Verification items for the finished model (mm, model axes). A direction names the side the tool comes from. Coordinates: 2 decimals unless noted, no trailing zeros. Order: outer loops, then holes, each group sorted by start corner. A loop starts at its lowest first (then second) coordinate and runs counter-clockwise, first axis right, second up. Notation, with made-up numbers: M 75.5,85.25 L 100.5,85.25 A19 ccw 100.5,109.25 Z; hole C -7.75,89 d2. An arc over 180 degrees is marked long. Answer as a JSON object with one key per item and string values. Group by question number.
(1) Gauge pin test, flat ends, axial feed: pin 1 Ø1 at (y, z) = (11.5, 4.5) entering from -X; pin 2 Ø3 at (x, z) = (0, 10) entering from +Y; pin 3 Ø6 at (x, y) = (-15.5, 15.5) entering from -Z; pin 4 Ø6 at (y, z) = (5.5, 11) entering from +X. Record the tip position at first contact, or that the pin passes through.
(2) Mould release check, pull along Z, two halves, no side actions. Record for faces 1 (the face through (-5, -12, 20)), 2 (the face through (14, -17, 7.5)), 3 (the face through (19.2, 0.4, 8.4)), 4 (the face through (17.07, -16.15, 13.84)): released by +Z, released by -Z, zero draft, split by the parting line, or undercut.
(3) Access from +Z, -Z, +X, -X, +Y, -Y to the whole of each face (thin tool, end or side, straight path). Record for faces 5 (the face through (0, -20, 2)), 6 (the face through (-0.4, 19.4, 11.6)).
(4) Cross-section at B-B (z = 10). Enter the section's corners in (x, y).
(5) Material ranges on line 1 (Z direction, x = 22.25, y = 0); line 2 (Y direction, x = -15, z = 15.75); line 3 (Y direction, x = -15.5, z = 11.75), recorded low to high.
(6) Cross-section at A-A (x = 0). Enter the section's corners in (y, z), plus the area to 3 significant figures.
(7) Cross-section at C-C (x = -6). Enter the section's corners in (y, z), plus the area to 3 significant figures.
(8) Cross-section at D-D (z = 15.75). Enter the section's corners in (x, y).
from build123d import *

# Parameters (mm, degrees)
SKETCH1_W                                           = 26
SKETCH1_H                                           = 20
F_2_CLEARANCE_HOLE1_D                               = 2.5
F_2_CLEARANCE_HOLE1_DEPTH                           = 6
HOLE1_D                                             = 25.4
HOLE1_DEPTH                                         = 20
HOLE1_CBORE_D                                       = 40
HOLE1_CBORE_DEPTH                                   = 3.4
F_4_CLEARANCE_HOLE1_D                               = 3.3
F_4_CLEARANCE_HOLE1_DEPTH                           = 65.407641206
F_4_CLEARANCE_HOLE2_D                               = 3.3
F_4_CLEARANCE_HOLE2_DEPTH                           = 13.407641206
F_4_CLEARANCE_HOLE3_D                               = 3.3
F_4_CLEARANCE_HOLE3_DEPTH                           = 13.407641206
CBORE_FOR_4_BINDING_HEAD_MACHINE_SCREW1_D           = 3.4
CBORE_FOR_4_BINDING_HEAD_MACHINE_SCREW1_DEPTH       = 20
CBORE_FOR_4_BINDING_HEAD_MACHINE_SCREW1_CBORE_D     = 6.5
CBORE_FOR_4_BINDING_HEAD_MACHINE_SCREW1_CBORE_DEPTH = 7.5


with BuildPart() as part:
    # Sketch1 → Revolve1 (revolve)
    with BuildSketch(Plane.XZ):
        with Locations((13, 10)):
            Rectangle(SKETCH1_W, SKETCH1_H)
    revolve(axis=Axis((0, 0, 20), (0, 0, -1)))

    # #2 Clearance Hole1
    with Locations(Plane(origin=(0, 0, 0), x_dir=(-1, 0, 0), z_dir=(0, 0, -1))):
        with Locations((-22.776165581, 3.200981322)):
            Hole(F_2_CLEARANCE_HOLE1_D / 2, depth=F_2_CLEARANCE_HOLE1_DEPTH)

    # Hole1
    with Locations(Plane(origin=(0, 0, 0), x_dir=(-1, 0, 0), z_dir=(0, 0, -1))):
        with Locations((0, 0)):
            CounterBoreHole(HOLE1_D / 2, HOLE1_CBORE_D / 2, HOLE1_CBORE_DEPTH, depth=HOLE1_DEPTH)

    # #4 Clearance Hole1
    with Locations(Plane(origin=(26, 0, 10), x_dir=(0, 1, 0), z_dir=(1, 0, 0))):
        with Locations((0, 0)):
            Hole(F_4_CLEARANCE_HOLE1_D / 2, depth=F_4_CLEARANCE_HOLE1_DEPTH)

    # #4 Clearance Hole2
    with Locations(Plane(origin=(0, 12.592358794, 0), x_dir=(-1, 0, 0), z_dir=(0, -1, 0))):
        with Locations((0, -10)):
            Hole(F_4_CLEARANCE_HOLE2_D / 2, depth=F_4_CLEARANCE_HOLE2_DEPTH)

    # #4 Clearance Hole3
    with Locations(Plane(origin=(0, -12.592358794, 0), x_dir=(1, 0, 0), z_dir=(0, 1, 0))):
        with Locations((0, -10)):
            Hole(F_4_CLEARANCE_HOLE3_D / 2, depth=F_4_CLEARANCE_HOLE3_DEPTH)

    # CBORE for #4 Binding Head Machine Screw1
    with Locations(Plane(origin=(0, 0, 0), x_dir=(-1, 0, 0), z_dir=(0, 0, -1))):
        with Locations((-15.5, -15.5), (15.5, -15.5), (15.5, 15.5), (-15.5, 15.5)):
            CounterBoreHole(CBORE_FOR_4_BINDING_HEAD_MACHINE_SCREW1_D / 2, CBORE_FOR_4_BINDING_HEAD_MACHINE_SCREW1_CBORE_D / 2, CBORE_FOR_4_BINDING_HEAD_MACHINE_SCREW1_CBORE_DEPTH, depth=CBORE_FOR_4_BINDING_HEAD_MACHINE_SCREW1_DEPTH)


solid = part.part
Taken from the geometry:
{
 "1": {"pin 1": "stops at x = -23.56", "pin 2": "passes through", "pin 3": "stops at z = 7.5", "pin 4": "stops at x = 25.88"},
 "2": {"face 1": "released by +Z", "face 2": "released by -Z", "face 3": "undercut", "face 4": "zero draft"},
 "3": {"face 5": "-Z", "face 6": "+Y, -Y"},
 "4": {"outline": "M -25.95,-1.65 A26 ccw -1.65,-25.95 L -1.65,-12.59 A12.7 cw -12.59,-1.65 Z; M -25.95,1.65 L -12.59,1.65 A12.7 cw -1.65,12.59 L -1.65,25.95 A26 ccw Z; M 1.65,-25.95 A26 ccw 25.95,-1.65 L 12.59,-1.65 A12.7 cw 1.65,-12.59 Z; M 1.65,12.59 A12.7 cw 12.59,1.65 L 25.95,1.65 A26 ccw 1.65,25.95 Z; hole C -15.5,-15.5 d3.4; hole C -15.5,15.5 d3.4; hole C 15.5,-15.5 d3.4; hole C 15.5,15.5 d3.4"},
 "5": {"line 1": "z = 0 to 8.35, 11.65 to 20", "line 2": "y = -21.24 to -17.12, -13.88 to 13.88, 17.12 to 21.24", "line 3": "y = -20.87 to -17.2, -13.8 to 13.8, 17.2 to 20.87"},
 "6": {"outline": "M -26,0 L -20,0 L -20,3.4 L -12.7,3.4 L -12.7,8.35 L -26,8.35 Z; M -26,11.65 L -12.7,11.65 L -12.7,20 L -26,20 Z; M 12.7,3.4 L 20,3.4 L 20,0 L 26,0 L 26,8.35 L 12.7,8.35 Z; M 12.7,11.65 L 26,11.65 L 26,20 L 12.7,20 Z", "area": "395 mm²"},
 "7": {"outline": "M -25.3,0 L -19.08,0 L -19.08,3.4 L -11.19,3.4 L -11.19,20 L -25.3,20 Z; M 11.19,3.4 L 19.08,3.4 L 19.08,0 L 25.3,0 L 25.3,20 L 11.19,20 Z", "area": "511 mm²"},
 "8": {"outline": "C 0,0 d52; hole C -15.5,-15.5 d3.4; hole C -15.5,15.5 d3.4; hole C 0,0 d25.4; hole C 15.5,-15.5 d3.4; hole C 15.5,15.5 d3.4"}
}
